Part model, mm, in its own coordinate system. A direction names the side the tool comes from. Give positions to 0.01 mm unless a question says otherwise; leave off trailing zeros. Loops run counter-clockwise (first coordinate to the right, second up) from the corner with the lowest first, then second, coordinate; pieces in that order, holes last. Notation, with made-up numbers: M 41,-23 L 71,-23 A18 ccw 71,-8 Z; hole C 42.5,-13 d9. An arc over 180 degrees is marked long. Answer in a Markdown table with one row per item.
from build123d import *

# Parameters (mm, degrees)
SKETCH_W       = 40
SKETCH_H       = 40
SKETCH_W_2     = 34
SKETCH_H_2     = 34
PAD_DEPTH      = 22.5
FILLET_R       = 3
FILLET001_R    = 3
FILLET002_R    = 3
FILLET003_R    = 3
SKETCH001_R    = 3
HOLE_DEPTH     = 23.197418
HOLE_TIPS_R    = 3
SKETCH002_R    = 3
HOLE001_DEPTH  = 23.197418
HOLE001_TIPS_R = 3


with BuildPart() as part:
    # Sketch → Pad (new body, symmetric)
    with BuildSketch(Plane.XY):
        Rectangle(SKETCH_W, SKETCH_H)
        Rectangle(SKETCH_W_2, SKETCH_H_2, mode=Mode.SUBTRACT)
    extrude(amount=PAD_DEPTH, both=True)

    # Fillet
    fillet_edges = [part.edges().sort_by_distance(p)[0] for p in [
        (-20, -20, 0),
    ]]
    fillet(fillet_edges, radius=FILLET_R)

    # Fillet001
    fillet001_edges = [part.edges().sort_by_distance(p)[0] for p in [
        (20, -20, 0),
    ]]
    fillet(fillet001_edges, radius=FILLET001_R)

    # Fillet002
    fillet002_edges = [part.edges().sort_by_distance(p)[0] for p in [
        (20, 20, 0),
    ]]
    fillet(fillet002_edges, radius=FILLET002_R)

    # Fillet003
    fillet003_edges = [part.edges().sort_by_distance(p)[0] for p in [
        (-20, 20, 0),
    ]]
    fillet(fillet003_edges, radius=FILLET003_R)

    # Sketch001 (on Face2 of Fillet003) → Hole (cut)
    with BuildSketch(Plane(origin=(0, 20, 0), x_dir=(-1, 0, 0), z_dir=(0, 1, 0))):
        Circle(SKETCH001_R)
    extrude(amount=-HOLE_DEPTH, mode=Mode.SUBTRACT)

    # Hole tips → Hole tip 1 section 0
    with BuildSketch(Plane(origin=(0, -3.197418, 0), x_dir=(-1, 0, 0), z_dir=(0, 1, 0)), mode=Mode.PRIVATE) as hole_tip_1_s0:
        Circle(HOLE_TIPS_R)
    loft([hole_tip_1_s0.sketch, Vertex(0, -5, 0)], mode=Mode.SUBTRACT)

    # Sketch002 (on Face9 of Hole) → Hole001 (cut)
    with BuildSketch(Plane.XZ.offset(20)):
        Circle(SKETCH002_R)
    extrude(amount=-HOLE001_DEPTH, mode=Mode.SUBTRACT)

    # Hole001 tips → Hole001 tip 1 section 0
    with BuildSketch(Plane.XZ.offset(-3.197418), mode=Mode.PRIVATE) as hole001_tip_1_s0:
        Circle(HOLE001_TIPS_R)
    loft([hole001_tip_1_s0.sketch, Vertex(0, 5, 0)], mode=Mode.SUBTRACT)


solid = part.part
(1) Pin check, flat tip, straight feed: pin 1 Ø8 at (x, y) = (-13.5, -8) entering from -Z. Stop position of the tip, or through.
Recorded:
| item | result |
|---|---|
| pin 1 | stops at z = -22.5 |
(2) Saw through at D-D (z = 0). Write the cut outline in (x, y), plus the area to 3 significant figures.
Recorded:
| item | result |
|---|---|
| outline | M -20,-17 A3 ccw -17,-20 L -3,-20 L -3,-17 L -17,-17 L -17,17 L -3,17 L -3,20 L -17,20 A3 ccw -20,17 Z; M 3,-20 L 17,-20 A3 ccw 20,-17 L 20,17 A3 ccw 17,20 L 3,20 L 3,17 L 17,17 L 17,-17 L 3,-17 Z |
| area | 400 mm^2 |
(3) Saw through at A-A (y = 3.5). Write the cut outline in (x, z).
Recorded:
| item | result |
|---|---|
| outline | M -20,-22.5 L -17,-22.5 L -17,22.5 L -20,22.5 Z; M 17,-22.5 L 20,-22.5 L 20,22.5 L 17,22.5 Z |
(4) Which spindle directions (+Z, -Z, +X, -X, +Y, -Y) get a long thin tool onto all of the face, cutting with end or side? Do faces 5 (the face through (17, 0, 0)), 6 (the face through (-4, -20, 0)). Say none if no direction does.
Recorded:
| item | result |
|---|---|
| face 5 | +Z, -Z |
| face 6 | +Z, -Z, +X, -X, -Y |
(5) Drill centre lines: line 1 along X through (y, z) = (-8, 1); line 2 along Z through (x, y) = (0, 18.7). Where is each one in solid material? Low to high.
Recorded:
| item | result |
|---|---|
| line 1 | x = -20 to -17, 17 to 20 |
| line 2 | z = -22.5 to -3, 3 to 22.5 |
(6) Pull direction Y, two halves, no side cores. Call faces 1 (the face through (-4, 17, 0)), 2 (the face through (-4, -17, 0)), 3 (the face through (-3, -19, 0)), 4 (the face through (-19.1, 19.14, -0.32)): +Y half, -Y half, draft (parallel to the pull), parting line (faces both ways), or undercut.
Recorded:
| item | result |
|---|---|
| face 1 | undercut |
| face 2 | undercut |
| face 3 | draft |
| face 4 | +Y half |
(7) Saw through at B-B (x = 0). Write the cut outline in (y, z), plus the area to 3 significant figures.
Recorded:
| item | result |
|---|---|
| outline | M -20,-22.5 L -17,-22.5 L -17,-3 L -20,-3 Z; M -20,3 L -17,3 L -17,22.5 L -20,22.5 Z; M 17,-22.5 L 20,-22.5 L 20,-3 L 17,-3 Z; M 17,3 L 20,3 L 20,22.5 L 17,22.5 Z |
| area | 234 mm^2 |
